```python
from build123d import *

# Parameters (mm, degrees)
SKETCH_1_W          = 40
SKETCH_1_H          = 40
EXTRUDE_1_DEPTH     = 33.5
SKETCH_2_W          = 45
SKETCH_2_H          = 45
EXTRUDE_2_DEPTH     = 7
SKETCH_3_R          = 20
CUT_EXTRUDE_3_DEPTH = 5
SKETCH_4_R          = 2.5
CUT_EXTRUDE_4_DEPTH = 15


with BuildPart() as part:
    # Эскиз1 → Бобышка-Вытянуть1 (new body)
    with BuildSketch(Plane.XY):
        Rectangle(SKETCH_1_W, SKETCH_1_H)
    extrude(amount=EXTRUDE_1_DEPTH)

    # Эскиз2 → Бобышка-Вытянуть2 (add)
    with BuildSketch(Plane.XY.offset(33.5)):
        Rectangle(SKETCH_2_W, SKETCH_2_H)
    extrude(amount=-EXTRUDE_2_DEPTH)

    # Эскиз3 → Вырез-Вытянуть3 (cut)
    with BuildSketch(Plane.XY.offset(33.5)):
        Circle(SKETCH_3_R)
    extrude(amount=-CUT_EXTRUDE_3_DEPTH, mode=Mode.SUBTRACT)

    # Эскиз4 → Вырез-Вытянуть4 (cut)
    with BuildSketch(Plane.XY.offset(28.5)):
        with Locations((-10.5, 0)):
            Circle(SKETCH_4_R)
        with Locations(Location((10.5, 0, 0), (0, 0, 180))):
            Circle(SKETCH_4_R)
    extrude(amount=-CUT_EXTRUDE_4_DEPTH, mode=Mode.SUBTRACT)


solid = part.part
```
The listing builds one solid part. Answer for the finished solid, in the listing's coordinates (mm). A direction names the side the tool comes from. Give positions to 0.01 mm unless a question says otherwise; leave off trailing zeros. Loops run counter-clockwise (first coordinate to the right, second up) from the corner with the lowest first, then second, coordinate; pieces in that order, holes last. Notation, with made-up numbers: (62, 15.25) - (82, 15.25) arc R18 cw to (82, 35.25) - close; hole circle Ø10 at (-20, 34.5). An arc over 180 degrees is marked (long way). Return JSON: item names as keys, results as strings. Group by question number.
1. Find section B-B (x = 0). Write down the section's boundary in (y, z), then the cut area to 4 significant figures.
2. Find section D-D (z = 4). Write down the section's boundary in (x, y).
3. Find section A-A (y = -16). Write down the section's boundary in (x, z).
4. Find section C-C (z = 23). Write down the section's boundary in (x, y), then the cut area to 3 significant figures.
5. Given pin 1 Ø4 at (x, y) = (8, -12) entering from -Z; pin 2 Ø5.5 at (x, y) = (-10, 1) entering from +Z; pin 3 Ø8 at (y, z) = (-14.5, 9) entering from +X; pin 4 Ø13 at (x, z) = (-7.5, 17.5) entering from -Y, each flat-ended and moving along its own axis, determine where each tip first touches the part or whether it passes through.
6. Determine the mould class of faces 1 (the flat face through (-20, 0, 13)), 2 (the flat face through (-11, 0, 13.5)), 3 (the flat face through (0, -20, 13)) for opening direction Y: pulls with the +Y half, pulls with the -Y half, needs draft (parallel to the pull), parting line crosses it, or undercut.
7. Which of the six approach directions +Z, -Z, +X, -X, +Y, -Y give full straight-line access (tool end or side, diameter ignored) to faces 4 (the flat face through (0, 20, 13)), 5 (the flat face through (20, 0, 13)), 6 (the cylindrical face through (13, 0, 21))?
8. Straight lines are drawn through the part: line 1 (Y direction, x = 10.5, z = 19.5); line 2 (Y direction, x = 0, z = 32.2); line 3 (X direction, y = 1, z = 20.5). For each, find the intervals that lie inside material, in ascending order. Write a range as [from, to].
Verdict:
{
 "1": {"outline": "(-22.5, 26.5) - (-20, 26.5) - (-20, 0) - (20, 0) - (20, 26.5) - (22.5, 26.5) - (22.5, 33.5) - (20, 33.5) - (20, 28.5) - (-20, 28.5) - (-20, 33.5) - (-22.5, 33.5) - close", "area": "1,175 mm^2"},
 "2": {"outline": "(-20, -20) - (20, -20) - (20, 20) - (-20, 20) - close"},
 "3": {"outline": "(-22.5, 26.5) - (-20, 26.5) - (-20, 0) - (20, 0) - (20, 26.5) - (22.5, 26.5) - (22.5, 33.5) - (12, 33.5) - (12, 28.5) - (-12, 28.5) - (-12, 33.5) - (-22.5, 33.5) - close"},
 "4": {"outline": "(-20, -20) - (20, -20) - (20, 20) - (-20, 20) - close; hole circle Ø5 at (-10.5, 0); hole circle Ø5 at (10.5, 0)", "area": "1,560 mm^2"},
 "5": {"pin 1": "stops at z = 0", "pin 2": "stops at z = 28.5", "pin 3": "stops at x = 20", "pin 4": "stops at y = -20"},
 "6": {"face 1": "needs draft", "face 2": "undercut", "face 3": "pulls with the -Y half"},
 "7": {"face 4": "-Z, +X, -X, +Y", "face 5": "-Z, +X, +Y, -Y", "face 6": "+Z"},
 "8": {"line 1": "y = [-20, -2.5], [2.5, 20]", "line 2": "y = [-22.5, -20], [20, 22.5]", "line 3": "x = [-20, -12.79], [-8.21, 8.21], [12.79, 20]"}
}
